Part model, mm, in its own coordinate system. Give positions to 0.01 mm unless a question says otherwise; leave off trailing zeros. Order: outer loops, then holes, each group sorted by start corner. A loop starts at its lowest first (then second) coordinate and runs counter-clockwise, first axis right, second up. Notation, with made-up numbers: M 77.25,-10.5 L 134.25,-10.5 A18 ccw 134.25,14.5 Z; hole C 71.5,45 d5. An arc over 180 degrees is marked long. Write each question's results on one line, items separated by ' | '. Start each with the question number.
from build123d import *

# Parameters (mm, degrees)
PAD_DEPTH    = 8.5
SKETCH001_W  = 0.5
SKETCH001_H  = 0.25
PAD001_DEPTH = 4.61


with BuildPart() as part:
    # Sketch → Pad (new body)
    with BuildSketch(Plane.XZ):
        Polygon((-5.29, 0), (-5.8, 0), (-5.8, 10.4), (5.8, 10.4), (5.8, 0), (5.29, 0), (5.29, 0.51), (-5.29, 0.51), align=None)
    extrude(amount=PAD_DEPTH)

    # Sketch001 → Pad001 (new body)
    with BuildSketch(Plane(origin=(0, 0, 0.51), x_dir=(1, 0, 0), z_dir=(0, 0, -1))):
        with Locations((-2.59, 2.125)):
            Rectangle(SKETCH001_W, SKETCH001_H)
        with Locations((0, 2.125)):
            Rectangle(SKETCH001_W, SKETCH001_H)
        with Locations((2.59, 2.125)):
            Rectangle(SKETCH001_W, SKETCH001_H)
    extrude(amount=PAD001_DEPTH)


solid = part.part
(1) Probe L1, parallel to Z at x = -1.25, y = -7. List the from-to ranges inside material, lowest first.
(2) Saw through at C-C on x = 4.75. Give the cut face in (y, z), plus the area to 3 significant figures.
(3) Saw through at A-A on z = -1.5. Give the cut face in (x, y), plus the area to 3 significant figures.
(4) Pull direction X, two halves, no side cores. Call faces 1 (the flat face through (5.8, -4, 5)), 2 (the flat face through (0, -8.5, 5)), 3 (the flat face through (0, -4, 0.51)), 4 (the flat face through (-5.8, -4, 5)): +X half, -X half, draft (parallel to the pull), parting line (faces both ways), or undercut.
(5) Drop flat-ended pins along their axis: P1, Ø0.6, axis at x = -2.5, z = -2.5, coming from the -Y side; P2, Ø0.6, axis at x = -5.5, y = -3.5, coming from the -Z side. Give the stop position or say it passes through.
(6) Saw through at B-B on y = -1.75. Give the cut face in (x, z), plus the area to 3 significant figures.
Taken from the geometry:
1) L1: z = 0.51 to 10.4
2) outline: M -8.5,0.51 L 0,0.51 L 0,10.4 L -8.5,10.4 Z | area: 84.1 mm²
3) outline: M -2.84,-2.25 L -2.34,-2.25 L -2.34,-2 L -2.84,-2 Z; M -0.25,-2.25 L 0.25,-2.25 L 0.25,-2 L -0.25,-2 Z; M 2.34,-2.25 L 2.84,-2.25 L 2.84,-2 L 2.34,-2 Z | area: 0.375 mm²
4) face 1: +X half | face 2: draft | face 3: undercut | face 4: -X half
5) P1: stops at y = -2.25 | P2: stops at z = 0
6) outline: M -5.8,0 L -5.29,0 L -5.29,0.51 L 5.29,0.51 L 5.29,0 L 5.8,0 L 5.8,10.4 L -5.8,10.4 Z | area: 115 mm²
